Verification items for this drawing (mm, ordinates from the low corner). A direction names the side the tool comes from. Round coordinates to 2 decimals unless told otherwise and drop trailing zeros. Write each loop counter-clockwise with the first axis right and the second up, starting at its lowest first coordinate (ties: lowest second). Pieces come first, ordered by that corner, then holes. Notation, with made-up numbers: M -12.75,28.25 L 13.25,28.25 A15 ccw 13.25,56.25 Z; hole C -14,31.5 d10. An arc over 180 degrees is marked long. One line per question, with ' | ' between items. Start each with the question number.
Q1. Release check for a two-part mould opening along Y. For the marked faces 1, 2 and 3 record: released by +Y, released by -Y, zero draft, split by the parting line, or undercut.
Q2. Gauge pin test, flat ends, axial feed: pin 1 (6 mm diameter, centred on x = 10.5, z = 3, fed in from +Y); pin 2 (6 mm diameter, centred on x = 40, y = 21, fed in from +Z). Record the tip position at first contact, or that the pin passes through.
Q3. Cross-section at D-D (z = 1.75). Record the boundary of the cut face in (x, y).
Q4. Cross-section at C-C (x = 25). Record the boundary of the cut face in (y, z), then the cut area to 3 significant figures.
Q5. Tool access check on the marked faces 4 and 5. Record the directions out of +Z, -Z, +X, -X, +Y, -Y that give a thin tool (end or side, any length) a straight path to the whole face; none if there is none.
Q6. Cross-section at A-A (z = 10.75). Record the boundary of the cut face in (x, y), then the cut area to 3 significant figures.
Q7. Cross-section at B-B (y = 32). Record the boundary of the cut face in (x, z).
Q8. Thickness scan on line 1 along Y through (x, z) = (25, 8.75); line 2 along Y through (x, z) = (25, 3.75); line 3 along X through (y, z) = (7, 2.75). Record the ranges inside material, lowest first. Write a range as from..to.
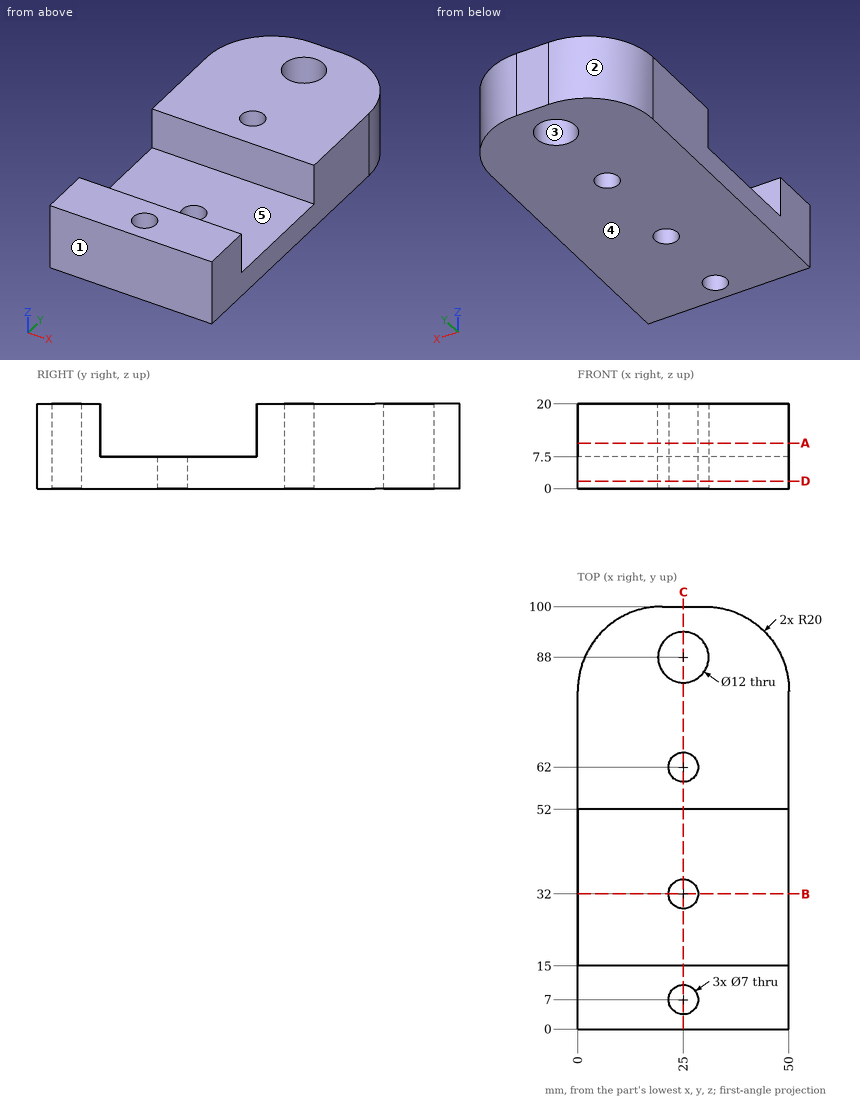
Determined:
1) face 1: released by -Y | face 2: released by +Y | face 3: undercut
2) pin 1: stops at y = 98.91 | pin 2: stops at z = 7.5
3) outline: M 0,0 L 50,0 L 50,80 A20 ccw 30,100 L 20,100 A20 ccw 0,80 Z; hole C 25,88 d12; hole C 25,7 d7; hole C 25,32 d7; hole C 25,62 d7
4) outline: M 0,0 L 3.5,0 L 3.5,20 L 0,20 Z; M 10.5,0 L 28.5,0 L 28.5,7.5 L 15,7.5 L 15,20 L 10.5,20 Z; M 35.5,0 L 58.5,0 L 58.5,20 L 52,20 L 52,7.5 L 35.5,7.5 Z; M 65.5,0 L 82,0 L 82,20 L 65.5,20 Z; M 94,0 L 100,0 L 100,20 L 94,20 Z | area: 965 mm²
5) face 4: -Z, +X, -X, +Y, -Y | face 5: +Z, +X, -X
6) outline: M 0,0 L 50,0 L 50,15 L 0,15 Z; M 0,52 L 50,52 L 50,80 A20 ccw 30,100 L 20,100 A20 ccw 0,80 Z; hole C 25,88 d12; hole C 25,7 d7; hole C 25,62 d7 | area: 2,790 mm²
7) outline: M 0,0 L 21.5,0 L 21.5,7.5 L 0,7.5 Z; M 28.5,0 L 50,0 L 50,7.5 L 28.5,7.5 Z
8) line 1: y = 0..3.5, 10.5..15, 52..58.5, 65.5..82, 94..100 | line 2: y = 0..3.5, 10.5..28.5, 35.5..58.5, 65.5..82, 94..100 | line 3: x = 0..21.5, 28.5..50
